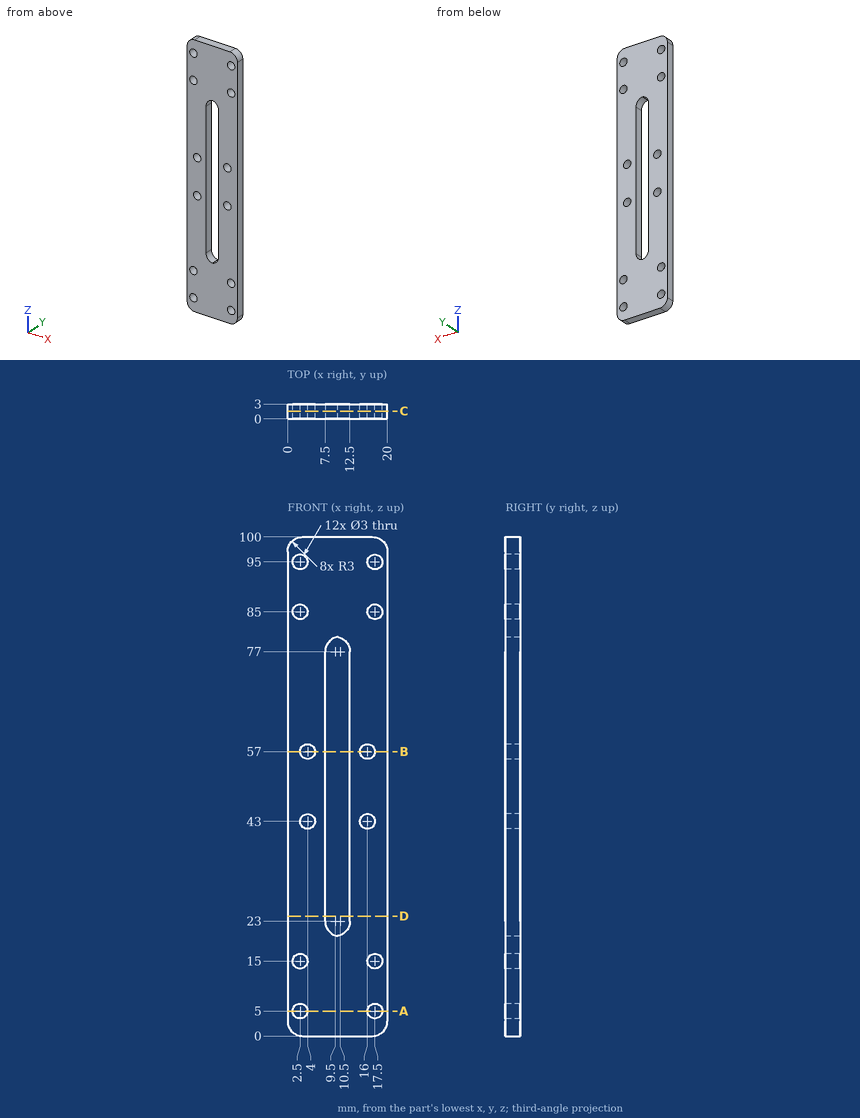
For this review, use the dimensioned drawing (mm, ordinates from the lowest corner) and the shaded views. Coordinates: 2 decimals unless noted, no trailing zeros. Loops run counter-clockwise (first coordinate to the right, second up) from the corner with the lowest first, then second, coordinate; pieces in that order, holes last. Notation, with made-up numbers: (28.5, 53) - (66.5, 53) arc R14 ccw to (66.5, 67) - close; hole circle Ø9 at (44.5, 24). An arc over 180 degrees is marked (long way). Use one line per item in the form item = value. Start each with the question number.
1) To check wall thickness, follow probe 1 along X at (y, z) = (1.7, 95); probe 2 along X at (y, z) = (2.15, 57); probe 3 along Z at (x, y) = (4.25, 2.6). State the ranges of each line that lie inside material, in increasing order. Write a range as from..to.
2) For pin 1 (1.8 mm diameter, centred on x = 17.5, z = 85, fed in from +Y), flat-tipped, find the tip position at first contact; note if it passes through.
3) Take a section at A-A (z = 5). State the section outline as (x, y) points.
4) Take a section at C-C (y = 1.55). State how many separate pieces and enclosed holes the cut face has, plus the area to 3 significant figures.
5) Take a section at B-B (z = 57). State the section outline as (x, y) points.
6) Take a section at D-D (z = 24). State the section outline as (x, y) points.
From the geometry:
q1.probe_1 = 0..1, 4..16, 19..20
q1.probe_2 = 0..2.5, 5.5..7.5, 12.5..14.5, 17.5..20
q1.probe_3 = 0..41.52, 44.48..55.52, 58.48..100
q2.pin_1 = through
q3.outline = (0, 0) - (1, 0) - (1, 3) - (0, 3) - close; (4, 0) - (16, 0) - (16, 3) - (4, 3) - close; (19, 0) - (20, 0) - (20, 3) - (19, 3) - close
q4.separate_pieces = 1
q4.enclosed_holes = 13
q4.area = 1,620 mm2
q5.outline = (0, 0) - (2.5, 0) - (2.5, 3) - (0, 3) - close; (5.5, 0) - (7.5, 0) - (7.5, 3) - (5.5, 3) - close; (12.5, 0) - (14.5, 0) - (14.5, 3) - (12.5, 3) - close; (17.5, 0) - (20, 0) - (20, 3) - (17.5, 3) - close
q6.outline = (0, 0) - (7.5, 0) - (7.5, 3) - (0, 3) - close; (12.5, 0) - (20, 0) - (20, 3) - (12.5, 3) - close
